The listing builds one solid part. Answer for the finished solid, in the listing's coordinates (mm). A direction names the side the tool comes from. Coordinates: 2 decimals unless noted, no trailing zeros. Write each loop counter-clockwise with the first axis right and the second up, starting at its lowest first coordinate (ties: lowest second). Pieces come first, ordered by that corner, then holes. Notation, with made-up numbers: M 61,67.5 L 97,67.5 A31 cw 97,92.5 Z; hole C -5,-23.5 d6. An arc over 180 degrees is marked long. Answer as CSV lines item,"result".
```python
from build123d import *

# Parameters (mm, degrees)
F0_W           = 410
F0_H           = 150
F1_DEPTH       = 5
F1_DEPTH_BACK  = 20
F2_R           = 45
F3_R           = 45
F4_R           = 45
F5_W           = 101.2708619237
F5_H           = 20.8901241422
F6_DEPTH       = 5
F6_DEPTH_BACK  = 20
F7_T1_DEPTH    = 25
F8_T1_DEPTH    = 25
F10_T          = -7
F12_R          = 4
F13_DEPTH      = 55.5
F14_W          = 329.6116441488
F14_H          = 83.0728560686
F15_DEPTH      = 25
F15_DEPTH_BACK = 25
F16_R          = 20
F20_D          = 3
F20_DEPTH      = 20
F20_TIP        = 0.9012909285


# Not quite as in the source:
# - a fillet or chamfer that OpenCascade refuses, or shapes differently, is made with other operations: its cross-section is extruded or revolved along the edge and cut away or added


with BuildPart() as f1:
    # F0 (on Front) → F1 (new body, two sides)
    with BuildSketch(Plane.XZ) as f1_sk:
        Rectangle(F0_W, F0_H)
    extrude(amount=F1_DEPTH)
    extrude(f1_sk.sketch, amount=-F1_DEPTH_BACK)

    # F2
    f2_edges = [f1.edges().sort_by_distance(p)[0] for p in [
        (-205, 7.5, 75),
        (-205, 7.5, -75),
    ]]
    fillet(f2_edges, radius=F2_R)

    # F3
    f3_edges = [f1.edges().sort_by_distance(p)[0] for p in [
        (205, 7.5, 75),
    ]]
    fillet(f3_edges, radius=F3_R)

    # F4
    f4_edges = [f1.edges().sort_by_distance(p)[0] for p in [
        (205, 7.5, -75),
    ]]
    fillet(f4_edges, radius=F4_R)

    # F5 (on Front) → F6 (join, two sides)
    with BuildSketch(Plane.XZ) as f6_sk:
        with Locations((-0.6414987147, -73.9290080965)):
            Rectangle(F5_W, F5_H)
    extrude(amount=F6_DEPTH)
    extrude(f6_sk.sketch, amount=-F6_DEPTH_BACK)

    # F7: fillet of radius 10 on 1 edges, made by hand

    # F7_s2 → F7_t1 (join)
    with BuildSketch(Plane.XZ.offset(-20)):
        with BuildLine():
            ThreePointArc((-61.2573210439, -75), (-54.4111286103, -77.7109912085), (-51.2769296765, -84.3740701675))
            Line((-51.2769296765, -84.3740701675), (-51.2769296765, -75))
            Line((-51.2769296765, -75), (-61.2573210439, -75))
        make_face()
    extrude(amount=F7_T1_DEPTH)

    # F8: fillet of radius 10 on 1 edges, made by hand

    # F8_s2 → F8_t1 (join)
    with BuildSketch(Plane.XZ.offset(-20)):
        with BuildLine():
            ThreePointArc((49.9939322472, -84.3740701675), (53.1281311809, -77.7109912085), (59.9743236145, -75))
            Line((59.9743236145, -75), (49.9939322472, -75))
            Line((49.9939322472, -75), (49.9939322472, -84.3740701675))
        make_face()
    extrude(amount=F8_T1_DEPTH)

    # F10
    f10_openings = [f1.faces().sort_by_distance(p)[0] for p in [
        (-0.010473, 20, -1.299239),
    ]]
    offset(amount=F10_T, openings=f10_openings)

    # F12 (on offset) → F13 (join)
    with BuildSketch(Plane.XZ.offset(3)):
        with Locations((-184.3019276857, 36.01404652)):
            Circle(F12_R)
        with Locations((-184.2796504498, -49.4647398591)):
            Circle(F12_R)
        with Locations((-36.0691249371, 51.8314018846)):
            Circle(F12_R)
        with Locations((-49.5743155479, 31.3860401511)):
            Circle(F12_R)
        with Locations((34.2704169452, 51.8314018846)):
            Circle(F12_R)
        with Locations((49.4637563825, 31.7611843348)):
            Circle(F12_R)
        with Locations((185.4535341263, 36.2629145384)):
            Circle(F12_R)
        with Locations((185.6411099434, -49.4575425982)):
            Circle(F12_R)
    extrude(amount=-F13_DEPTH)

    # F14 (on face) → F15 (cut, two sides)
    with BuildSketch(Plane.XZ) as f15_sk:
        with Locations((2.6797705796, -19.8723953217)):
            Rectangle(F14_W, F14_H)
    extrude(amount=F15_DEPTH, mode=Mode.SUBTRACT)
    extrude(f15_sk.sketch, amount=-F15_DEPTH_BACK, mode=Mode.SUBTRACT)

    # F16
    f16_edges = [f1.edges().sort_by_distance(p)[0] for p in [
        (-162.126051, -1.5, 21.664033),
        (167.485593, -1.5, 21.664033),
        (167.485593, -1.5, -61.408823),
        (-162.126051, -1.5, -61.408823),
    ]]
    fillet(f16_edges, radius=F16_R)

    # F20
    with Locations(Plane.XZ.offset(5)):
        with Locations((-184.4574809074, 54.7145232558), (-184.4574809074, -54.8582747579), (185.6484860182, -54.8582747579), (185.6484860182, 54.7145232558)):
            Hole(F20_D / 2, depth=F20_DEPTH)
            with Locations((0, 0, -(F20_DEPTH + F20_TIP / 2))):  # 118° drill point
                Cone(0, F20_D / 2, F20_TIP, mode=Mode.SUBTRACT)


solid = f1.part
```
Q1. Straight lines are drawn through the part: line 1 (Z direction, x = 31, y = 8); line 2 (Z direction, x = 144.5, y = 9); line 3 (X direction, y = -1, z = -16). For each, find the intervals that lie inside material, in ascending order.
Output:
line 1,"-84.37 to -77.37, 49.53 to 54.13, 68 to 75"
line 2,"-75 to -68, 68 to 75"
line 3,"-205 to -162.13, 167.49 to 205"
Q2. Find section C-C (y = 48.5). Give the vertices of the cut face in (x, z).
Output:
outline,"C -184.3,36.01 d8; C -184.28,-49.46 d8; C -49.57,31.39 d8; C -36.07,51.83 d8; C 34.27,51.83 d8; C 49.46,31.76 d8; C 185.45,36.26 d8; C 185.64,-49.46 d8"
Q3. Find section A-A (x = -85). Give the vertices of the cut face in (y, z).
Output:
outline,"M -5,-75 L 20,-75 L 20,-68 L 2,-68 L 2,-61.41 L -5,-61.41 Z; M -5,21.66 L 2,21.66 L 2,68 L 20,68 L 20,75 L -5,75 Z"
Q4. Find section B-B (z = -3.5). Give the vertices of the cut face in (x, y), and give its area (3 significant figures).
Output:
outline,"M -205,-5 L -162.13,-5 L -162.13,2 L -198,2 L -198,20 L -205,20 Z; M 167.49,-5 L 205,-5 L 205,20 L 198,20 L 198,2 L 167.49,2 Z"
area,"815 mm2"
Q5. The mould has two halves that part along X. Classify faces 1 (the flat face through (-3, -5, 32)), 2 (the cylindrical face through (-192.168, 7.675, 61.468)), 3 (the flat face through (109, 11, -68)): pulls with the +X half, pulls with the -X half, needs draft (parallel to the pull), parting line crosses it, or undercut.
Output:
face 1,"needs draft"
face 2,"pulls with the -X half"
face 3,"undercut"
Q6. For faces 4 (the cylindrical face through (-156.42, -1.45, 15.65)), 5 (the flat face through (-36, 52.5, 52)), 6 (the cylindrical face through (-188.3, 26.9, 36.19)), determine the directions among +Z, -Z, +X, -X, +Y, -Y from which every point of the face is accessible in a straight line to the end or side of a thin tool.
Output:
face 4,"+Y, -Y"
face 5,"+Z, -Z, +X, -X, +Y"
face 6,"+Y"
Q7. Flat-ended cylindrical pins translate along their axes: pin 1 Ø3 at (y, z) = (21, 41) entering from -X; pin 2 Ø4 at (x, z) = (-184.46, 54.71) entering from +Y; pin 3 Ø5.5 at (x, y) = (54, 14) entering from -Z. Find the tip coordinate at first contact, or state that the pin passes through.
Output:
pin 1,"x = -203.9"
pin 2,"y = 2"
pin 3,"z = -80.11"
